The figure shows three views and two pictorial views of one solid part (mm, origin at its lowest corner). Answer the questions. A direction names the side the tool comes from. Round coordinates to 2 decimals unless told otherwise and drop trailing zeros. Write each loop counter-clockwise with the first axis right and the second up, starting at its lowest first coordinate (ties: lowest second). Pieces come first, ordered by that corner, then holes. Notation, with made-up numbers: M 69.5,80 L 78.5,80 A11 cw 78.5,89 Z; hole C -39.75,-36 d7. An arc over 180 degrees is marked long. Answer in a Markdown table with one row per item.
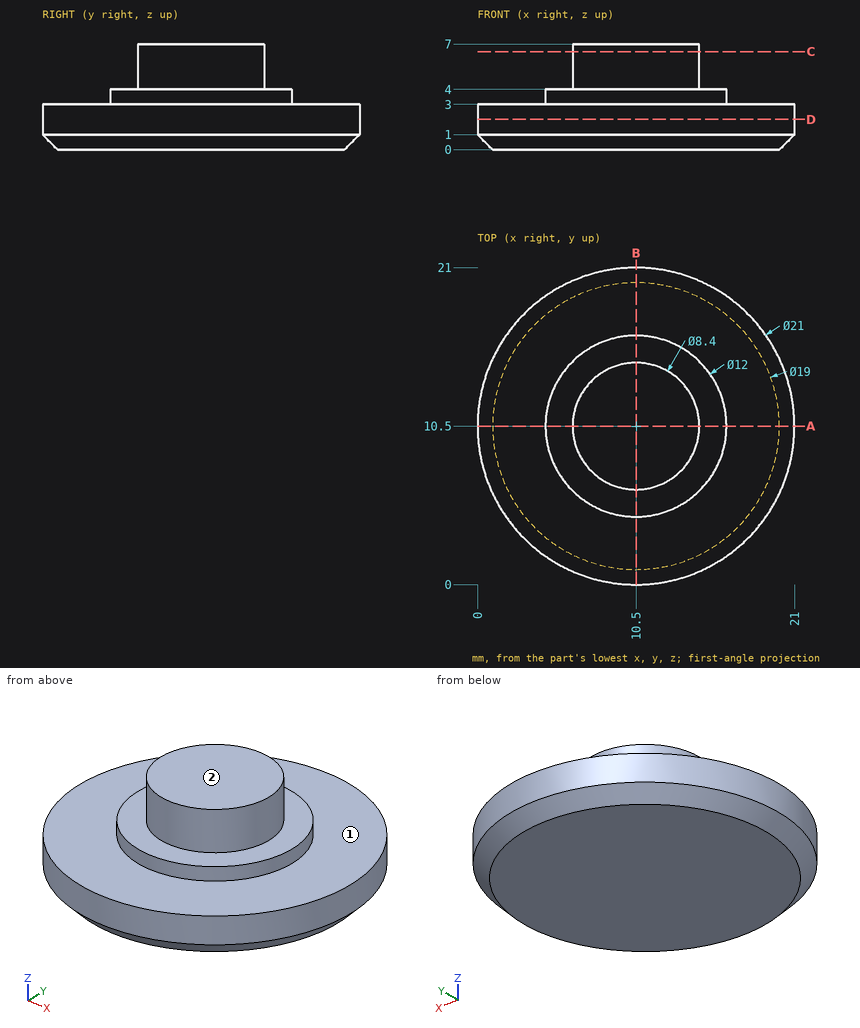
1. A tool of negligible diameter and unlimited length cuts with its end or side. For the marked faces 1 and 2, from which of +Z, -Z, +X, -X, +Y, -Y can it reach the whole face along a straight path? Write none if from no direction.
Calculated:
| item | result |
|---|---|
| face 1 | +Z |
| face 2 | +Z, +X, -X, +Y, -Y |
2. The part is cut by section C-C (z = 6.5). Determine the outline of the cut face in (x, y), plus the area to 3 significant figures.
Calculated:
| item | result |
|---|---|
| outline | C 10.5,10.5 d8.4 |
| area | 55.4 mm² |
3. The part is cut by section D-D (z = 2). Determine the outline of the cut face in (x, y), plus the area to 3 significant figures.
Calculated:
| item | result |
|---|---|
| outline | C 10.5,10.5 d21 |
| area | 346 mm² |
4. Given pin 1 (1.5 mm diameter, centred on x = 13, z = 6, fed in from -Y), flat-ended and moving along its own axis, determine where the tip first touches the part or whether it passes through.
Calculated:
| item | result |
|---|---|
| pin 1 | stops at y = 6.68 |
5. Consider line 1 along Z through (x, y) = (9.5, 16.75); line 2 along Z through (x, y) = (14.25, 14.5); line 3 along X through (y, z) = (5.25, 2). Determine where each line is inside the solid, lowest interval first. Write a range as from..to.
Calculated:
| item | result |
|---|---|
| line 1 | z = 0..3 |
| line 2 | z = 0..4 |
| line 3 | x = 1.41..19.59 |
6. The part is cut by section A-A (y = 10.5). Determine the outline of the cut face in (x, z), plus the area to 3 significant figures.
Calculated:
| item | result |
|---|---|
| outline | M 0,1 L 1,0 L 20,0 L 21,1 L 21,3 L 16.5,3 L 16.5,4 L 14.7,4 L 14.7,7 L 6.3,7 L 6.3,4 L 4.5,4 L 4.5,3 L 0,3 Z |
| area | 99.2 mm² |
